Design review of the part built by this model. Coordinates are the model's own, in mm. Coordinates: 2 decimals unless noted, no trailing zeros. Loops run counter-clockwise (first coordinate to the right, second up) from the corner with the lowest first, then second, coordinate; pieces in that order, holes last.
Q1. Wall thickness on probe 1 along X at (y, z) = (21.5, 2.85); probe 2 along X at (y, z) = (38.5, 0.65); probe 3 along Y at (x, z) = (1.5, 0.2): over which ranges is each line inside the solid? List them lowest first.
Q2. Add section A-A on y = 34. Give the boundary of the cut face in (x, z) (3 decimals).
Q3. Add section C-C on z = 1.15. Give the boundary of the cut face in (x, y), and give its area (3 significant figures).
Q4. Add section B-B on x = 0. Give the boundary of the cut face in (y, z) (3 decimals), and give its area (3 significant figures).
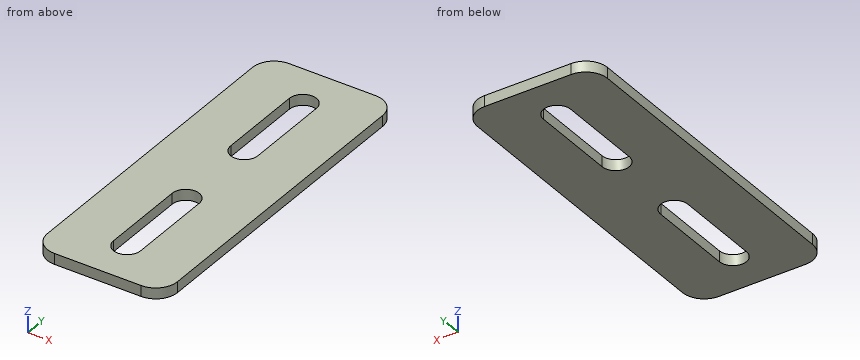
```python
from build123d import *

# Parameters (mm, degrees)
SKETCH1_W           = 38.1
SKETCH1_H           = 101.6
BOSS_EXTRUDE1_DEPTH = 3.175
FILLET1_R           = 6.35
CUT_EXTRUDE1_DEPTH  = 55.34724579


with BuildPart() as part:
    # Sketch1 → Boss-Extrude1 (new body)
    with BuildSketch(Plane.XY):
        Rectangle(SKETCH1_W, SKETCH1_H)
    extrude(amount=BOSS_EXTRUDE1_DEPTH)

    # Fillet1
    fillet1_edges = [part.edges().sort_by_distance(p)[0] for p in [
        (19.05, -50.8, 1.5875),
        (-19.05, -50.8, 1.5875),
        (-19.05, 50.8, 1.5875),
        (19.05, 50.8, 1.5875),
    ]]
    fillet(fillet1_edges, radius=FILLET1_R)

    # Sketch2 → Cut-Extrude1 (cut, through all)
    with BuildSketch(Plane.XY.offset(3.175)):
        with BuildLine():
            Line((3.96875, 38.1), (3.96875, 12.7))
            ThreePointArc((3.96875, 12.7), (0, 8.73125), (-3.96875, 12.7))
            Line((-3.96875, 12.7), (-3.96875, 38.1))
            ThreePointArc((-3.96875, 38.1), (0, 42.06875), (3.96875, 38.1))
        make_face()
        with BuildLine():
            Line((3.96875, -12.7), (3.96875, -38.1))
            ThreePointArc((3.96875, -38.1), (0, -42.06875), (-3.96875, -38.1))
            Line((-3.96875, -38.1), (-3.96875, -12.7))
            ThreePointArc((-3.96875, -12.7), (0, -8.73125), (3.96875, -12.7))
        make_face()
    extrude(amount=-CUT_EXTRUDE1_DEPTH, mode=Mode.SUBTRACT)


solid = part.part
```
Entries:
1. probe 1: x = -19.05 to -3.97, 3.97 to 19.05
1. probe 2: x = -19.05 to -3.95, 3.95 to 19.05
1. probe 3: y = -50.8 to -41.77, -9.03 to 9.03, 41.77 to 50.8
2. outline: (-19.05, 0) - (-3.969, 0) - (-3.969, 3.175) - (-19.05, 3.175) - close; (3.969, 0) - (19.05, 0) - (19.05, 3.175) - (3.969, 3.175) - close
3. outline: (-19.05, -44.45) arc R6.35 ccw to (-12.7, -50.8) - (12.7, -50.8) arc R6.35 ccw to (19.05, -44.45) - (19.05, 44.45) arc R6.35 ccw to (12.7, 50.8) - (-12.7, 50.8) arc R6.35 ccw to (-19.05, 44.45) - close; hole (-3.97, -38.1) arc R3.97 ccw to (3.97, -38.1) - (3.97, -12.7) arc R3.97 ccw to (-3.97, -12.7) - close; hole (-3.97, 12.7) arc R3.97 ccw to (3.97, 12.7) - (3.97, 38.1) arc R3.97 ccw to (-3.97, 38.1) - close
3. area: 3,330 mm2
4. outline: (-50.8, 0) - (-42.069, 0) - (-42.069, 3.175) - (-50.8, 3.175) - close; (-8.731, 0) - (8.731, 0) - (8.731, 3.175) - (-8.731, 3.175) - close; (42.069, 0) - (50.8, 0) - (50.8, 3.175) - (42.069, 3.175) - close
4. area: 111 mm2
